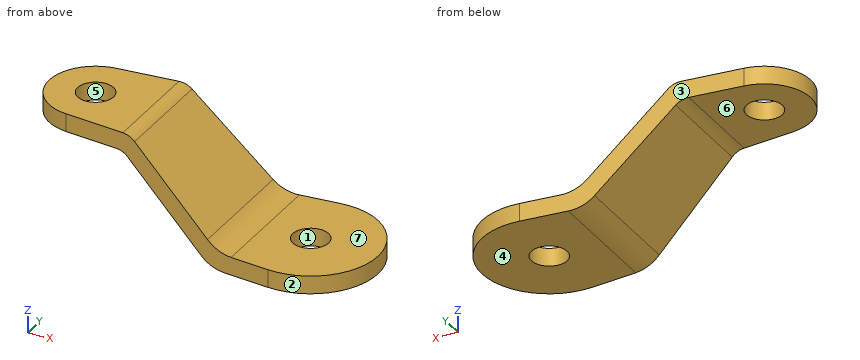
Autodesk Inventor part; units mm, degrees
ref_plane "SideProfilePlane" through (0, 12, 0) normal (0, 1, 0) x (-1, 0, 0)
ref_plane "YZ Plane" through (0, 0, 0) normal (1, 0, 0) x (0, 1, 0)
ref_plane "XY Plane" through (0, 0, 0) normal (0, 0, 1) x (1, 0, 0)
sketch "Body" plane through (0, 0, 0) normal (0, 0, 1) x (1, 0, 0)
  circle A0 centre (0, 0) radius 7.75
  line L0 (0, 0) -> (36, 0) construction
  circle A1 centre (36, 0) radius 11.25
  line L1 (-0.7535, 7.7133) -> (34.9062, 11.1967)
  line L2 (-0.7535, -7.7133) -> (34.9062, -11.1967)
  dimension "SmallDiameter" = 15.5
  dimension "d1" = 36
  dimension "LargeDiameter" = 22.5
extrude "BodyFeature" add sketch "Body" along normal blind 18
sketch "Sketch2" plane through (0, 0, 18) normal (0, 0, 1) x (1, 0, 0)
  arc A0 (-0.7535, 7.7133) -> (-0.7535, -7.7133) centre (0, 0) ccw construction
  line L0 (-0.7535, -7.7133) -> (34.9062, -11.1967) construction
  arc A1 (34.9062, -11.1967) -> (34.9062, 11.1967) centre (36, 0) ccw construction
  line L1 (34.9062, 11.1967) -> (-0.7535, 7.7133) construction
hole "BodyHolesFeature" at (0, 0, 18) at (36, 0, 18) direction (0, 0, -1) diameter 6 end through all
ref_plane "SideProfilePlane" through (0, 12, 0) normal (0, 1, 0) x (-1, 0, 0)
sketch "SideProfile" plane through (0, 12, 0) normal (0, 1, 0) x (-1, 0, 0)
  line L0 (7.75, 18) -> (0.7535, 18) construction
  line L1 (7.75, 18) -> (7.75, 15)
  line L2 (7.75, 15) -> (-9.25, 15)
  line L3 (-9.25, 15) -> (-24.75, 0)
  line L4 (-24.75, 0) -> (-47.25, 0)
  line L5 (-34.9062, 0) -> (0.7535, 0) construction
  line L6 (-47.25, 0) -> (-47.25, 18) construction
  line L7 (-34.9062, 18) -> (-47.25, 18) construction
  line L8 (-34.9062, 18) -> (0.7535, 18) construction
  line L9 (-25.9639, 3) -> (-10.4639, 18)
  line L10 (-47.25, 3) -> (-25.9639, 3)
  line L11 (-47.25, 0) -> (-47.25, 3)
  line L12 (7.75, 18) -> (-10.4639, 18)
  dimension "Thickness" = 3
  dimension "d15" = 3
  dimension "d16" = 3
  dimension "d17" = 17
  dimension "d18" = 22.5
extrude "SideProfileFeature" cut sketch "SideProfile" against normal through all keep common part
fillet "SmallFilletFeature" radius 3 2 edges at (9.25, 0, 15) (10.4639, 0, 18)
fillet "LargeFilletFeature" radius 6 2 edges at (24.75, 0, 0) (25.9639, 0, 3)
equation "\"d15\" = Thickness"
equation "\"d16\" = Thickness"
equation "\"d18\" = LargeDiameter"
properties part number "BackConnector"
CAD build for the part. Positions are in the model's coordinates, mm. Face numbers are marked on the shaded views. A direction names the side the tool comes from. Round coordinates to 2 decimals unless told otherwise and drop trailing zeros. Loops run counter-clockwise (first coordinate to the right, second up) from the corner with the lowest first, then second, coordinate; pieces in that order, holes last. Notation, with made-up numbers: M -9,62 L -2,62 A19 ccw -2,84 Z; hole C -5.75,20.5 d6. An arc over 180 degrees is marked long. One line per question, with ' | ' between items. Start each with the question number.
Item 1: Cut at B-B, the plane x = 36. Write the cut outline in (y, z).
Item 2: Cut at D-D, the plane z = 8.75. Write the cut outline in (x, y).
Item 3: Two-plate mould, pull along Y, no slides. Class the marked faces 1, 2, 3 and 4: pulls with the +Y half, pulls with the -Y half, needs draft (parallel to the pull), parting line crosses it, or undercut.
Item 4: Pin check, flat tips, straight feed: pin 1 Ø5 at (x, y) = (1.5, -5.5) entering from -Z; pin 2 Ø6 at (x, y) = (21, -5.5) entering from +Z; pin 3 Ø4 at (x, z) = (29, 6.5) entering from +Y; pin 4 Ø8 at (y, z) = (-6, 14.5) entering from +X. Stop position of each tip, or through.
Item 5: Cut at C-C, the plane y = -5.5. Write the cut outline in (x, z).
Item 6: Which spindle directions (+Z, -Z, +X, -X, +Y, -Y) get a long thin tool onto all of the face, cutting with end or side? Do the marked faces 5, 6 and 7. Say none if no direction does.
Item 7: Wall check: line 1 (Y direction, x = 0, z = 16.9); line 2 (X direction, y = 0, z = 17.1); line 3 (X direction, y = 0, z = 16.85). Give the ranges that are in metal, low to high.
Item 8: Cut at A-A, the plane y = 0. Write the cut outline in (x, z), plus the area to 3 significant figures.
Responses:
1) outline: M -11.25,0 L -3,0 L -3,3 L -11.25,3 Z; M 3,0 L 11.25,0 L 11.25,3 L 3,3 Z
2) outline: M 15.71,-9.32 L 20.02,-9.74 L 20.02,9.74 L 15.71,9.32 Z
3) face 1: undercut | face 2: parting line crosses it | face 3: pulls with the +Y half | face 4: needs draft
4) pin 1: stops at z = 15 | pin 2: stops at z = 10.71 | pin 3: passes through | pin 4: stops at x = 18.21
5) outline: M -5.46,15 L 8.04,15 A3 cw 10.12,14.16 L 23.01,1.69 A6 ccw 27.18,0 L 45.81,0 L 45.81,3 L 28.39,3 A6 cw 24.22,4.69 L 11.34,17.16 A3 ccw 9.25,18 L -5.46,18 Z
6) face 5: +Z, -Z | face 6: -Z, -X, +Y, -Y | face 7: +Z, +X, +Y, -Y
7) line 1: y = -7.79 to -3, 3 to 7.79 | line 2: x = -7.75 to -3, 3 to 11.39 | line 3: x = -7.75 to -3, 3 to 11.65
8) outline: M -7.75,15 L -3,15 L -3,18 L -7.75,18 Z; M 3,15 L 8.04,15 A3 cw 10.12,14.16 L 23.01,1.69 A6 ccw 27.18,0 L 33,0 L 33,3 L 28.39,3 A6 cw 24.22,4.69 L 11.34,17.16 A3 ccw 9.25,18 L 3,18 Z; M 39,0 L 47.25,0 L 47.25,3 L 39,3 Z | area: 147 mm²
